from build123d import *

# Parameters (mm, degrees)
SKETCH1_W               = 128
SKETCH1_H               = 86
BOSS_EXTRUDE1_DEPTH     = 3
CUT_EXTRUDE1_DEPTH      = 3
CUT_EXTRUDE2_DEPTH      = 3
CUT_EXTRUDE3_DEPTH      = 3
CUT_EXTRUDE4_DEPTH      = 3
SKETCH9_W               = 123
SKETCH9_H               = 42.35
CUT_EXTRUDE5_DEPTH      = 3
SKETCH23_W              = 13.2
SKETCH23_H              = 13.2
BOSS_EXTRUDE7_DEPTH     = 27
MIRROR2_COPY_1_SKETCH_W = 13.2
MIRROR2_COPY_1_SKETCH_H = 13.2
MIRROR2_COPY_1_DEPTH    = 27
SKETCH25_W              = 8.6
SKETCH25_H              = 7.1
BOSS_EXTRUDE8_DEPTH     = 3


with BuildPart() as part:
    # Sketch1 → Boss-Extrude1 (new body)
    with BuildSketch(Plane(origin=(0, 0, 0), x_dir=(1, 0, 0), z_dir=(0, 1, 0))):
        Rectangle(SKETCH1_W, SKETCH1_H)
    extrude(amount=BOSS_EXTRUDE1_DEPTH)

    # Sketch3 → Cut-Extrude1 (cut)
    with BuildSketch(Plane(origin=(0, 0, 0), x_dir=(-1, 0, 0), z_dir=(0, -1, 0))):
        Polygon((64, -43), (56.999376177, -43), (64, -35.995743323), align=None)
    extrude(amount=-CUT_EXTRUDE1_DEPTH, mode=Mode.SUBTRACT)

    # Sketch6 → Cut-Extrude2 (cut)
    with BuildSketch(Plane.XZ):
        Polygon((-64, -43), (-57, -43), (-64, -36.003281028), align=None)
    extrude(amount=-CUT_EXTRUDE2_DEPTH, mode=Mode.SUBTRACT)

    # Sketch7 → Cut-Extrude3 (cut)
    with BuildSketch(Plane.XZ):
        Polygon((64, 43), (57, 43), (64, 36), align=None)
    extrude(amount=-CUT_EXTRUDE3_DEPTH, mode=Mode.SUBTRACT)

    # Sketch8 → Cut-Extrude4 (cut)
    with BuildSketch(Plane.XZ):
        Polygon((64, -43), (64, -36), (57, -43), align=None)
    extrude(amount=-CUT_EXTRUDE4_DEPTH, mode=Mode.SUBTRACT)

    # Sketch9 → Cut-Extrude5 (cut)
    with BuildSketch(Plane.XZ):
        Rectangle(SKETCH9_W, SKETCH9_H)
    extrude(amount=-CUT_EXTRUDE5_DEPTH, mode=Mode.SUBTRACT)

    # Sketch23 → Boss-Extrude7 (add)
    with BuildSketch(Plane.XZ):
        with Locations((54.651250219, 31.000549)):
            Rectangle(SKETCH23_W, SKETCH23_H)
    boss_extrude7 = extrude(amount=BOSS_EXTRUDE7_DEPTH)

    # Mirror1: Boss-Extrude7 across plane
    add(boss_extrude7.mirror(Plane.XY))

    # Mirror2: Boss-Extrude7 across plane
    add(boss_extrude7.mirror(Plane(origin=(0, 0, 0), x_dir=(0, 0, 1), z_dir=(1, 0, 0))))

    # Mirror2 copy 1 sketch → Mirror2 copy 1 (add)
    with BuildSketch(Plane(origin=(0, 0, 0), x_dir=(-1, 0, 0), z_dir=(0, -1, 0))):
        with Locations((54.651250219, 31.000549)):
            Rectangle(MIRROR2_COPY_1_SKETCH_W, MIRROR2_COPY_1_SKETCH_H)
    extrude(amount=MIRROR2_COPY_1_DEPTH)

    # Sketch25 → Boss-Extrude8 (add)
    with BuildSketch(Plane.XZ):
        with Locations((-43.751250219, -28.035331383)):
            Rectangle(SKETCH25_W, SKETCH25_H)
    boss_extrude8 = extrude(amount=BOSS_EXTRUDE8_DEPTH)

    # Mirror4: Boss-Extrude8 across plane
    add(boss_extrude8.mirror(Plane.XY))


solid = part.part
Geometry check sheet. Reference: the model listing, model coordinates, mm. A direction names the side the tool comes from. Coordinates: 2 decimals unless noted, no trailing zeros. Loops run counter-clockwise (first coordinate to the right, second up) from the corner with the lowest first, then second, coordinate; pieces in that order, holes last. Notation, with made-up numbers: (-25.5, 81.25) - (-12.5, 81.25) arc R15 ccw to (-12.5, 107.25) - close; hole circle Ø11 at (39.25, 4.25). An arc over 180 degrees is marked (long way). Use one line per item in the form item = value. Start each with the question number.
Item 1: Section check B-B, the plane x = -54. Enter the section's corners in (y, z) (3 decimals), and give its area (3 significant figures).
Item 2: Section check D-D, the plane x = 38.5. Enter the section's corners in (y, z) (3 decimals).
Item 3: Tool access check on faces 1 (the face through (-44, -1, -31.585)), 2 (the face through (-61.5, 1, 0)), 3 (the face through (-44, -1, 31.585)), 4 (the face through (-55, -13, -37.601)), 5 (the face through (-55, -13, 24.401)). Record the directions out of +Z, -Z, +X, -X, +Y, -Y that give a thin tool (end or side, any length) a straight path to the whole face; none if there is none.
Item 4: Gauge pin test, flat ends, axial feed: pin 1 (6.5 mm diameter, centred on y = -11, z = -32.5, fed in from -X); pin 2 (6.5 mm diameter, centred on x = 55, y = -13.5, fed in from -Z); pin 3 (2 mm diameter, centred on y = -9, z = 21.5, fed in from +X); pin 4 (4 mm diameter, centred on x = 55.5, y = -16, fed in from +Z). Record the tip position at first contact, or that the pin passes through.
Item 5: Section check C-C, the plane y = -21.5. Enter the section's corners in (x, z), and give its area (3 significant figures).
Item 6: Mould release check, pull along X, two halves, no side actions. Record for faces 6 (the face through (60, 1, 40)), 7 (the face through (-39.451, -1, -28)), 8 (the face through (-55, -13, 37.601)): +X half, -X half, draft (parallel to the pull), parting line (faces both ways), or undercut.
Item 7: Section check A-A, the plane z = -7. Enter the section's corners in (x, y), and give its area (3 significant figures).
Item 8: Thickness scan on probe 1 along Z at (x, y) = (-51.5, -16.5); probe 2 along X at (y, z) = (-18, 33.5); probe 3 along Z at (x, y) = (9, 1.75) (3 decimals). Record the ranges inside material, lowest first.
Computed:
q1.outline = (-27, -37.601) - (0, -37.601) - (0, -43) - (3, -43) - (3, -21.175) - (0, -21.175) - (0, -24.401) - (-27, -24.401) - close; (-27, 24.401) - (0, 24.401) - (0, 21.175) - (3, 21.175) - (3, 43) - (0, 43) - (0, 37.601) - (-27, 37.601) - close
q1.area = 844 mm2
q2.outline = (0, -43) - (3, -43) - (3, -21.175) - (0, -21.175) - close; (0, 21.175) - (3, 21.175) - (3, 43) - (0, 43) - close
q3.face_1 = -Z, -Y
q3.face_2 = +Y, -Y
q3.face_3 = +Z, -Y
q3.face_4 = -Z, +X, -X, -Y
q3.face_5 = +X, -X, -Y
q4.pin_1 = -61.25
q4.pin_2 = -37.6
q4.pin_3 = through
q4.pin_4 = 37.6
q5.outline = (-61.25, -37.6) - (-48.05, -37.6) - (-48.05, -24.4) - (-61.25, -24.4) - close; (-61.25, 24.4) - (-48.05, 24.4) - (-48.05, 37.6) - (-61.25, 37.6) - close; (48.05, -37.6) - (61.25, -37.6) - (61.25, -24.4) - (48.05, -24.4) - close; (48.05, 24.4) - (61.25, 24.4) - (61.25, 37.6) - (48.05, 37.6) - close
q5.area = 697 mm2
q6.face_6 = +X half
q6.face_7 = undercut
q6.face_8 = draft
q7.outline = (-64, 0) - (-61.5, 0) - (-61.5, 3) - (-64, 3) - close; (61.5, 0) - (64, 0) - (64, 3) - (61.5, 3) - close
q7.area = 15.0 mm2
q8.probe_1 = -37.6 to -24.4, 24.4 to 37.6
q8.probe_2 = -61.25 to -48.05, 48.05 to 61.25
q8.probe_3 = -43 to -21.175, 21.175 to 43
